Could you check a few things on this drawing? It's one solid part, dimensions in mm from its lowest x, y, z. A direction names the side the tool comes from. Give positions to 0.01 mm unless a question says otherwise; leave off trailing zeros. Order: outer loops, then holes, each group sorted by start corner. A loop starts at its lowest first (then second) coordinate and runs counter-clockwise, first axis right, second up. Notation, with made-up numbers: M 47,19.25 L 62,19.25 A18 ccw 62,41.25 Z; hole C 77,34.25 d4. An arc over 180 degrees is marked long. One line per item, written item: value. Start each with the question number.
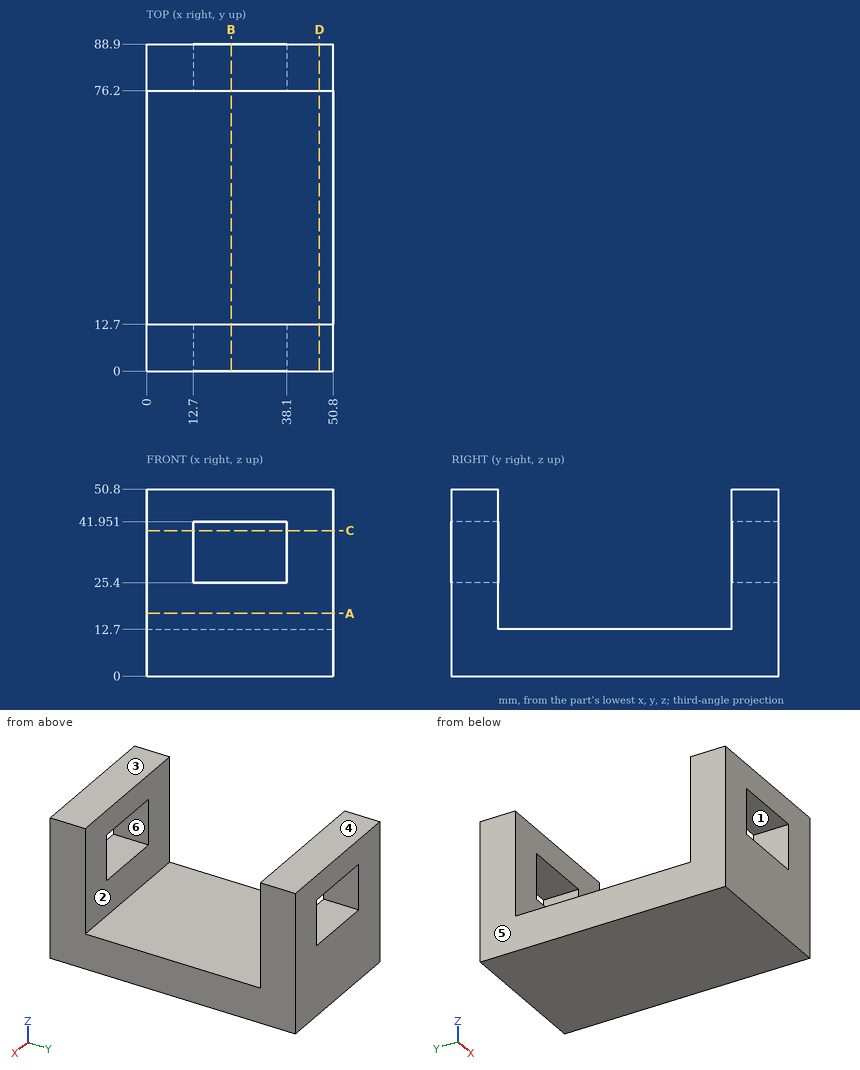
Item 1: I want a section at A-A on z = 17. Write out the boundary of the cut face in (x, y), plus the area to 3 significant figures.
Item 2: Will this pin go through, and if not, where does the flat tip stop? P1, Ø15, axis at x = 33.5, y = 58, coming from the +Z side.
Item 3: We'd pull the mould along X, two halves only. Please class the marked faces 4, 5 and 6: +X half, -X half, draft (parallel to the pull), parting line (faces both ways), or undercut.
Item 4: I want a section at D-D on x = 47. Write out the boundary of the cut face in (y, z), plus the area to 3 significant figures.
Item 5: I want a section at C-C on z = 39.5. Write out the boundary of the cut face in (x, y), plus the area to 3 significant figures.
Item 6: Please list where these lines run through material, in increasing order: probe 1 along Y at (x, z) = (4.5, 27); probe 2 along Z at (x, y) = (37, 12); probe 3 along X at (y, z) = (77, 41). Write a range as [from, to].
Item 7: For the marked faces 1, 2 and 3, which set-ups out of +Z, -Z, +X, -X, +Y, -Y let a thin tool reach every point of the face, with its end or its side?
Item 8: I want a section at B-B on x = 23. Write out the boundary of the cut face in (y, z), plus the area to 3 significant figures.
Answer below:
1. outline: M 0,0 L 50.8,0 L 50.8,12.7 L 0,12.7 Z; M 0,76.2 L 50.8,76.2 L 50.8,88.9 L 0,88.9 Z
1. area: 1,290 mm²
2. P1: stops at z = 12.7
3. face 4: draft
3. face 5: -X half
3. face 6: undercut
4. outline: M 0,0 L 88.9,0 L 88.9,50.8 L 76.2,50.8 L 76.2,12.7 L 12.7,12.7 L 12.7,50.8 L 0,50.8 Z
4. area: 2,100 mm²
5. outline: M 0,0 L 12.7,0 L 12.7,12.7 L 0,12.7 Z; M 0,76.2 L 12.7,76.2 L 12.7,88.9 L 0,88.9 Z; M 38.1,0 L 50.8,0 L 50.8,12.7 L 38.1,12.7 Z; M 38.1,76.2 L 50.8,76.2 L 50.8,88.9 L 38.1,88.9 Z
5. area: 645 mm²
6. probe 1: y = [0, 12.7], [76.2, 88.9]
6. probe 2: z = [0, 25.4], [41.95, 50.8]
6. probe 3: x = [0, 12.7], [38.1, 50.8]
7. face 1: +Y, -Y
7. face 2: +Z, +X, -X
7. face 3: +Z, +X, -X, +Y, -Y
8. outline: M 0,0 L 88.9,0 L 88.9,25.4 L 76.2,25.4 L 76.2,12.7 L 12.7,12.7 L 12.7,25.4 L 0,25.4 Z; M 0,41.95 L 12.7,41.95 L 12.7,50.8 L 0,50.8 Z; M 76.2,41.95 L 88.9,41.95 L 88.9,50.8 L 76.2,50.8 Z
8. area: 1,680 mm²
